from build123d import *

# Parameters (mm, degrees)
SKETCH2_R          = 6.25
CUT_EXTRUDE1_DEPTH = 7
CUT_EXTRUDE2_DEPTH = 4
FILLET1_R          = 5


with BuildPart() as part:
    # Sketch1 → Revolve1 (revolve)
    with BuildSketch(Plane(origin=(0, 0, 0), x_dir=(1, 0, 0), z_dir=(0, 1, 0))):
        Polygon((0, 0), (0, 10), (5.659340659, 10), (15, 0), align=None)
    revolve(axis=Axis((0, 0, 0), (0, 0, -1)))

    # Sketch2 → Cut-Extrude1 (cut)
    with BuildSketch(Plane.XY):
        Circle(SKETCH2_R)
        Polygon((2.989454216, 1.750189559), (-0.020981512, 3.464038074), (-3.010435727, 1.713848515), (-2.989454216, -1.750189559), (0.020981512, -3.464038074), (3.010435727, -1.713848515), align=None, mode=Mode.SUBTRACT)
    extrude(amount=-CUT_EXTRUDE1_DEPTH, mode=Mode.SUBTRACT)

    # Sketch4 → Cut-Extrude2 (cut)
    with BuildSketch(Plane.XY):
        Polygon((-0.020981512, 3.464038074), (-3.010435727, 1.713848515), (-2.989454216, -1.750189559), (0.020981512, -3.464038074), (3.010435727, -1.713848515), (2.989454216, 1.750189559), align=None)
    extrude(amount=-CUT_EXTRUDE2_DEPTH, mode=Mode.SUBTRACT)

    # Fillet1
    fillet1_edges = [part.edges().sort_by_distance(p)[0] for p in [
        (-5.659340659, 0, -10),
    ]]
    fillet(fillet1_edges, radius=FILLET1_R)


solid = part.part
Geometry: final body of the model. Coordinates: model frame, mm. A direction names the side the tool comes from. Coordinates: 2 decimals unless noted, no trailing zeros. Order: outer loops, then holes, each group sorted by start corner. A loop starts at its lowest first (then second) coordinate and runs counter-clockwise, first axis right, second up. Notation, with made-up numbers: (-17.75, 72.5) - (37.25, 72.5) arc R21 ccw to (37.25, 77.5) - close; hole circle Ø4 at (7, 9.5). An arc over 180 degrees is marked (long way). Use one line per item in the form item = value.
1) Section B-B (z = -3.5). Return loops of the section in (x, y), then the cut area to 3 significant figures.
Solutions:
outline = circle Ø23.46 at (0, 0); hole circle Ø12.5 at (0, 0)
area = 310 mm^2
2) Section A-A (z = -1.5). Return loops of the section in (x, y).
Solutions:
outline = circle Ø27.2 at (0, 0); hole circle Ø12.5 at (0, 0)
3) Ray query, L1, parallel to Y at x = 0, z = -5.5; L2, parallel to X at y = -1, z = -3; L3, parallel to Y at x = 0, z = -4.25. Return the intervals inside material, ascending.
Solutions:
L1 = -9.86 to -6.25, -3.45 to 3.45, 6.25 to 9.86
L2 = -12.16 to -6.17, 6.17 to 12.16
L3 = -11.03 to -6.25, -3.45 to 3.45, 6.25 to 11.03
4) Set-up query: faces 4 (the face through (0, 0, -10)), 5 (the face through (5.96, 1.88, -3.45)). Return all of +Z, -Z, +X, -X, +Y, -Y with unobstructed straight access to the full face (end or side cutting, diameter ignored); none if empty.
Solutions:
face_4 = -Z, +X, -X, +Y, -Y
face_5 = +Z
5) Pin query (flat end, axial travel): pin 1 (5 mm diameter, centred on x = 0.5, y = 0, fed in from +Z); pin 2 (1 mm diameter, centred on x = 4.5, y = 3.5, fed in from -Z); pin 3 (3 mm diameter, centred on x = 3, z = -6, fed in from -Y). Return the tip coordinate at first contact, or that it passes through.
Solutions:
pin_1 = -4
pin_2 = -9.7
pin_3 = -10.43
6) Mould query, pull axis Y, two halves, no side actions, for faces 1 (the face through (-0.2, 6.5, 0)), 2 (the face through (7.28, -2.29, -7.89)), 3 (the face through (1.5, -2.6, -5.5)). Classes: +Y half, -Y half, draft (parallel to the pull), parting line (faces both ways), or undercut.
Solutions:
face_1 = draft
face_2 = parting line
face_3 = undercut
